Input: dimensioned drawing with shaded views. Units: mm. Origin: part minimum x, y, z. Round coordinates to 2 decimals unless told otherwise and drop trailing zeros. Loops run counter-clockwise (first coordinate to the right, second up) from the corner with the lowest first, then second, coordinate; pieces in that order, holes last. Notation, with made-up numbers: (37, 58.25) - (92, 58.25) arc R10 ccw to (92, 72.25) - close; hole circle Ø6 at (-11, -18). An arc over 180 degrees is marked (long way). Answer as a JSON object with one key per item and string values. Group by question number.
Item 1: First-contact query: pin 1 (3.5 mm diameter, centred on x = 12.7, z = 44.45, fed in from -Y); pin 2 (6.5 mm diameter, centred on x = 12.7, z = 63.5, fed in from -Y). Flat tips, straight axial feed; report the tip coordinate or a pass-through.
Item 2: Line query: line 1 (Z direction, x = 12.7, y = 1.3); line 2 (Z direction, x = 14.5, y = 0.3) (1 decimal); line 3 (X direction, y = 0.2, z = 46). Output: solid intervals per line, ascending.
Item 3: Section C-C (x = 6.35). Return the cut outline in (y, z) (1 decimal).
Item 4: Section A-A (z = 63.5). Count the separate pieces of the cut face and the enclosed holes in it, plus the area to 3 significant figures.
Item 5: Section B-B (y = 0.7). Return the cut outline in (x, z).
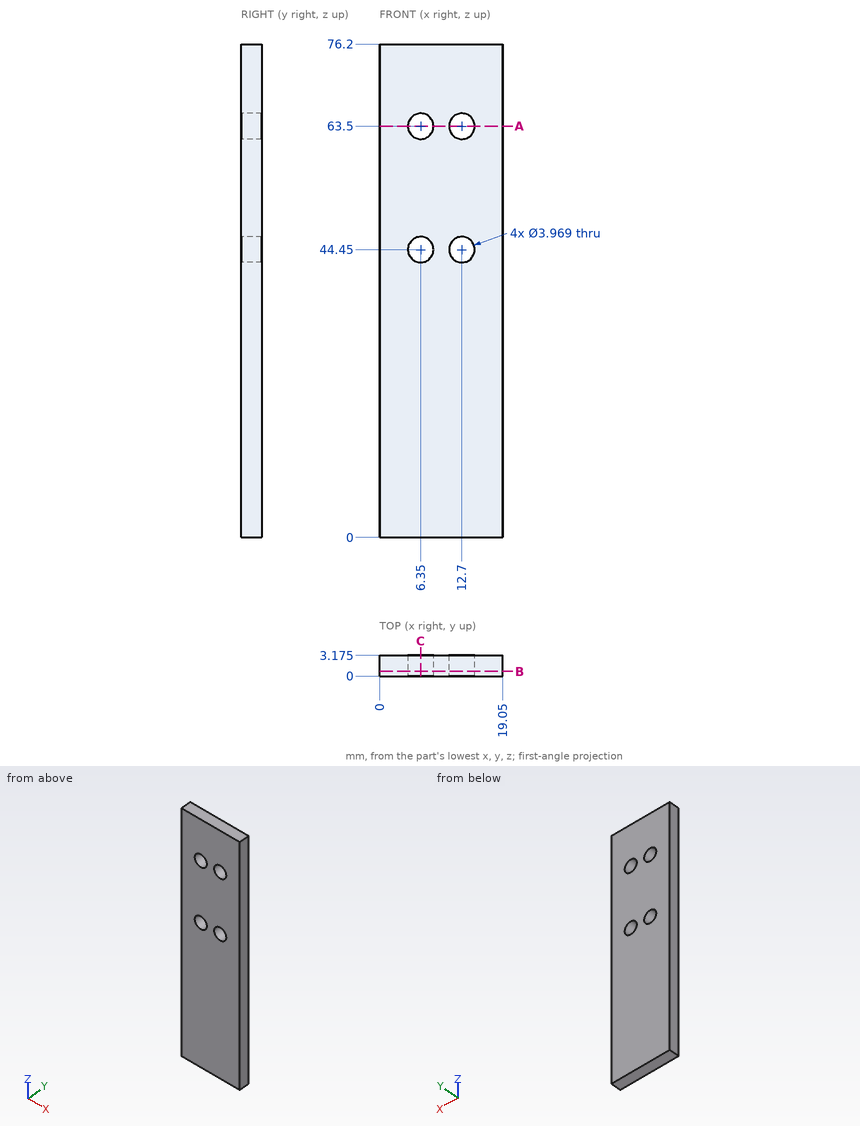
Values:
{
 "1": {"pin 1": "passes through", "pin 2": "stops at y = 0"},
 "2": {"line 1": "z = 0 to 42.47, 46.43 to 61.52, 65.48 to 76.2", "line 2": "z = 0 to 43.6, 45.3 to 62.7, 64.3 to 76.2", "line 3": "x = 0 to 5.11, 7.59 to 11.46, 13.94 to 19.05"},
 "3": {"outline": "(0, 0) - (3.2, 0) - (3.2, 42.5) - (0, 42.5) - close; (0, 46.4) - (3.2, 46.4) - (3.2, 61.5) - (0, 61.5) - close; (0, 65.5) - (3.2, 65.5) - (3.2, 76.2) - (0, 76.2) - close"},
 "4": {"separate pieces": "3", "enclosed holes": "0", "area": "35.3 mm^2"},
 "5": {"outline": "(0, 0) - (19.05, 0) - (19.05, 76.2) - (0, 76.2) - close; hole circle Ø3.97 at (6.35, 44.45); hole circle Ø3.97 at (6.35, 63.5); hole circle Ø3.97 at (12.7, 44.45); hole circle Ø3.97 at (12.7, 63.5)"}
}
